```python
from build123d import *

# Parameters (mm, degrees)
F1_DEPTH = 63.5
F0_W     = 25.4
F0_H     = 19.05
F2_DEPTH = 25.4
F3_DEPTH = 7.9375


with BuildPart() as f1:
    # F0 (on Front) → F1 (new body, symmetric)
    with BuildSketch(Plane.XZ):
        Polygon((22.225, 9.525), (-41.275, 9.525), (-41.275, -9.525), (41.275, -9.525), (41.275, 9.525), align=None)
    extrude(amount=F1_DEPTH, both=True)

    # F0 (on Front) → F2 (join, symmetric)
    with BuildSketch(Plane.XZ):
        with BuildLine():
            Line((22.225, 27.0002), (22.225, 9.525))
            Line((22.225, 9.525), (41.275, 9.525))
            Line((41.275, 9.525), (41.275, 27.0002))
            ThreePointArc((41.275, 27.0002), (45.9246798487, 38.2255201513), (57.15, 42.8752))
            Line((57.15, 42.8752), (60.325, 42.8752))
            Line((60.325, 42.8752), (60.325, 61.9252))
            Line((60.325, 61.9252), (57.15, 61.9252))
            add(Edge.make_bspline(
                [(54.5051235228, 61.8249075138), (55.3877284617, 61.8679154461), (56.2694699988, 61.9014230074), (57.15, 61.9252)],
                knots=[109.4292782466, 109.4292782466, 109.4292782466, 109.4292782466, 111.5045361635, 111.5045361635, 111.5045361635, 111.5045361635], degree=3))
            ThreePointArc((54.5051235228, 61.8249075138), (31.5362543156, 50.7423914957), (22.225, 27.0002))
        make_face()
        with Locations((73.025, 52.4002)):
            Rectangle(F0_W, F0_H)
    extrude(amount=F2_DEPTH, both=True)

    # F0 (on Front) → F3 (join, symmetric)
    with BuildSketch(Plane.XZ):
        with BuildLine():
            add(Edge.make_bspline(
                [(-41.275, 9.525), (-40.9758715935, 30.8734704245), (7.9649702933, 59.5570800062), (54.5051235228, 61.8249075138)],
                knots=[0, 0, 0, 0, 109.4292782466, 109.4292782466, 109.4292782466, 109.4292782466], degree=3))
            Line((-41.275, 9.525), (22.225, 9.525))
            Line((22.225, 9.525), (22.225, 27.0002))
            ThreePointArc((22.225, 27.0002), (31.5362543156, 50.7423914957), (54.5051235228, 61.8249075138))
        make_face()
    extrude(amount=F3_DEPTH, both=True)


solid = f1.part
```
Source: CAD feature listing. Evaluate the final solid. Frame: model axes, mm. A direction names the side the tool comes from. Coordinates: 2 decimals unless noted, no trailing zeros. Loops run counter-clockwise (first coordinate to the right, second up) from the corner with the lowest first, then second, coordinate; pieces in that order, holes last. Notation, with made-up numbers: M -34,83.5 L -11,83.5 A29 ccw -11,119.5 Z; hole C 72,62 d2. An arc over 180 degrees is marked long. Use a Markdown table: item, result. Add a question column.
Q1. Section query B-B, the plane x = 75. Return loops of the section in (y, z).
Q2. Section query A-A, the plane y = 32.5. Return loops of the section in (x, z) (3 decimals).
Q3. Material intervals for L1, parallel to Y at x = 20, z = 24; L2, parallel to Z at x = 72, y = 18; L3, parallel to Y at x = 64, z = 47, sorted ascending.
Q4. First-contact query: pin 1 (3 mm diameter, centred on x = 19, z = 26, fed in from -Y); pin 2 (5 mm diameter, centred on y = -22.5, z = 23, fed in from -X) (3 decimals); pin 3 (8 mm diameter, centred on y = 6, z = 5.5, fed in from +X) (3 decimals). Flat tips, straight axial feed; report the tip coordinate or a pass-through.
Q5. Access query for faces 1 (the cylindrical face through (31.786, 16.547, 51.009)), 2 (the flat face through (46, 25.4, 42)), 3 (the flat face through (71, 0, 42.875)), 4 (the flat face through (22.225, -17, 18)), 5 (the flat face through (46, -25.4, 42)). Directions: +Z, -Z, +X, -X, +Y, -Y. A direction counts if a zero-diameter tool reaches every point of the face in a straight line with its end or side. Return the directions, or none.
Result:
| question | item | result |
|---|---|---|
| 1 | outline | M -25.4,42.88 L 25.4,42.88 L 25.4,61.93 L -25.4,61.93 Z |
| 2 | outline | M -41.275,-9.525 L 41.275,-9.525 L 41.275,9.525 L -41.275,9.525 Z |
| 3 | L1 | y = -7.94 to 7.94 |
| 3 | L2 | z = 42.88 to 61.93 |
| 3 | L3 | y = -25.4 to 25.4 |
| 4 | pin 1 | stops at y = -7.94 |
| 4 | pin 2 | stops at x = 22.225 |
| 4 | pin 3 | stops at x = 41.275 |
| 5 | face 1 | +Z, -X, +Y |
| 5 | face 2 | +Z, +X, -X, +Y |
| 5 | face 3 | -Z, +X, +Y, -Y |
| 5 | face 4 | +Z, -X, -Y |
| 5 | face 5 | +Z, +X, -X, -Y |
